Check sheet for the modelled part. Datum: model origin and axes. Units: mm. Face numbers are marked on the shaded views. A direction names the side the tool comes from. Round coordinates to 2 decimals unless told otherwise and drop trailing zeros. Loops run counter-clockwise (first coordinate to the right, second up) from the corner with the lowest first, then second, coordinate; pieces in that order, holes last. Notation, with made-up numbers: (-37, -12) -> (-29, -12) arc R34 cw to (-29, 26) -> close; hole circle Ø8 at (35, -17.5). An arc over 180 degrees is marked (long way). Return JSON: item names as keys, results as strings.
from build123d import *

# Parameters (mm, degrees)
F0_R      = 21.6324082339
F1_DEPTH  = 50.8
F2_R      = 21.6324082339
F3_DEPTH  = 50.8
F4_W      = 43.638148787
F4_H      = 45.5662310123
F5_DEPTH  = 12.7
F6_R      = 21.6201983054
F7_DEPTH  = 12.7
F8_W      = 43.2470137948
F8_H      = 45.5075465143
F9_DEPTH  = 12.7
F10_R     = 21.600140632
F11_DEPTH = 12.7
F12_R     = 9.0838177262
F13_DEPTH = 101.601
F14_R     = 8.547587073
F15_DEPTH = 101.601


with BuildPart() as f1:
    # F0 (on Front) → F1 (new body)
    with BuildSketch(Plane.XZ):
        Circle(F0_R)
    extrude(amount=F1_DEPTH)

    # F2 (on face) → F3 (join)
    with BuildSketch(Plane(origin=(0, 0, 0), x_dir=(-1, 0, 0), z_dir=(0, 1, 0))):
        Circle(F2_R)
    extrude(amount=F3_DEPTH)

    # F4 (on face) → F5 (join)
    with BuildSketch(Plane.XZ.offset(50.8)):
        with Locations((0.1866661596, 22.7831155062)):
            Rectangle(F4_W, F4_H)
    extrude(amount=-F5_DEPTH)

    # F6 (on face) → F7 (join)
    with BuildSketch(Plane.XZ.offset(50.8)):
        with Locations((0.1866661596, 45.5662310123)):
            Circle(F6_R)
    extrude(amount=-F7_DEPTH)

    # F8 (on face) → F9 (join)
    with BuildSketch(Plane(origin=(0, 50.8, 0), x_dir=(-1, 0, 0), z_dir=(0, 1, 0))):
        with Locations((-0.0089013365, 22.7537732571)):
            Rectangle(F8_W, F8_H)
    extrude(amount=-F9_DEPTH)

    # F10 (on face) → F11 (join)
    with BuildSketch(Plane(origin=(0, 50.8, 0), x_dir=(-1, 0, 0), z_dir=(0, 1, 0))):
        with Locations((-0.0089013365, 45.5075465143)):
            Circle(F10_R)
    extrude(amount=-F11_DEPTH)

    # F12 (on face) → F13 (cut, through all)
    with BuildSketch(Plane.XZ.offset(50.8)):
        Circle(F12_R)
    extrude(amount=-F13_DEPTH, mode=Mode.SUBTRACT)

    # F14 (on face) → F15 (cut, through all)
    with BuildSketch(Plane.XZ.offset(50.8)):
        with Locations((0, 48.1973513961)):
            Circle(F14_R)
    extrude(amount=-F15_DEPTH, mode=Mode.SUBTRACT)


solid = f1.part
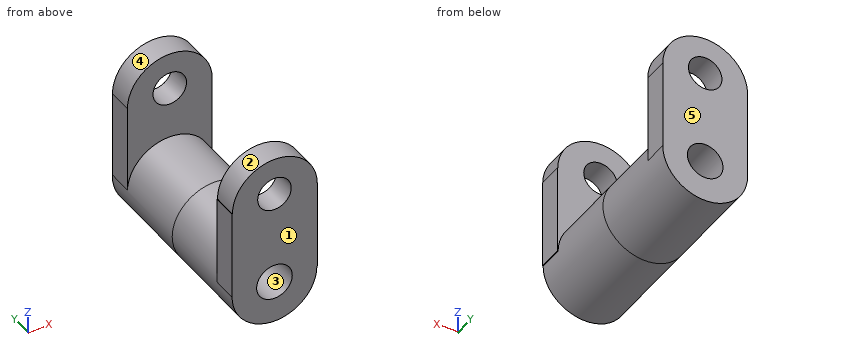
Q1. Draft check along Z on the marked faces 1, 2 and 3. Enter one of: released by +Z, released by -Z, zero draft, split by the parting line, or undercut.
Results list:
{"face 1": "zero draft", "face 2": "released by +Z", "face 3": "undercut"}
Q2. Material ranges on line 1 (Z direction, x = 0, y = 28); line 2 (Y direction, x = 11, z = 39); line 3 (Z direction, x = 0, y = -41), recorded low to high.
Results list:
{"line 1": "-21.63 to -9.08, 9.08 to 21.63", "line 2": "-50.8 to -38.1, 38.1 to 50.8", "line 3": "-21.63 to -9.08, 9.08 to 39.65, 56.74 to 67.19"}
Q3. Tool access check on the marked faces 4 and 5. Record the directions out of +Z, -Z, +X, -X, +Y, -Y that give a thin tool (end or side, any length) a straight path to the whole face; none if there is none.
Results list:
{"face 4": "+Z, +Y", "face 5": "+Z, -Z, +X, -X, +Y"}
Q4. Go/stop test with flat-tipped pins: pin 1 (2 mm diameter, centred on y = -7.5, z = -2, fed in from +X); pin 2 (14 mm diameter, centred on y = 45.5, z = 20.5, fed in from -X); pin 3 (2 mm diameter, centred on y = -9.5, z = 5, fed in from -X). Record where each tip stops, or that it passes through.
Results list:
{"pin 1": "x = 21.61", "pin 2": "x = -21.61", "pin 3": "x = -21.26"}
Q5. Section check B-B (z = 55). Record the boundary of the cut face in (x, y).
Results list:
{"outline": "(-19.39, 38.1) -> (-5.18, 38.1) -> (-5.18, 50.8) -> (-19.39, 50.8) -> close; (-19.27, -50.8) -> (-5.18, -50.8) -> (-5.18, -38.1) -> (-19.27, -38.1) -> close; (5.18, -50.8) -> (19.64, -50.8) -> (19.64, -38.1) -> (5.18, -38.1) -> close; (5.18, 38.1) -> (19.41, 38.1) -> (19.41, 50.8) -> (5.18, 50.8) -> close"}
Q6. Section check A-A (z = 27). Record the boundary of the cut face in (x, y).
Results list:
{"outline": "(-21.63, -50.8) -> (22.01, -50.8) -> (22.01, -38.1) -> (-21.63, -38.1) -> close; (-21.61, 38.1) -> (21.63, 38.1) -> (21.63, 50.8) -> (-21.61, 50.8) -> close"}
Q7. Section check D-D (y = 26). Record the boundary of the cut face in (x, z), then the cut area to 3 significant figures.
Results list:
{"outline": "circle Ø43.26 at (0, 0); hole circle Ø18.17 at (0, 0)", "area": "1,210 mm^2"}
Q8. Section check C-C (x = 0). Record the boundary of the cut face in (y, z), then the cut area to 3 significant figures.
Results list:
{"outline": "(-50.8, -21.63) -> (50.8, -21.63) -> (50.8, -9.08) -> (-50.8, -9.08) -> close; (-50.8, 9.08) -> (50.8, 9.08) -> (50.8, 39.65) -> (38.1, 39.65) -> (38.1, 21.63) -> (-38.1, 21.63) -> (-38.1, 39.65) -> (-50.8, 39.65) -> close; (-50.8, 56.74) -> (-38.1, 56.74) -> (-38.1, 67.19) -> (-50.8, 67.19) -> close; (38.1, 56.74) -> (50.8, 56.74) -> (50.8, 67.11) -> (38.1, 67.11) -> close", "area": "3,270 mm^2"}
